Autodesk Inventor part; units mm, degrees
ref_plane "YZ Plane" through (0, 0, 0) normal (1, 0, 0) x (0, 1, 0)
ref_plane "XZ Plane" through (0, 0, 0) normal (0, 1, 0) x (-1, 0, 0)
ref_plane "XY Plane" through (0, 0, 0) normal (0, 0, 1) x (1, 0, 0)
sketch "Sketch1" plane through (0, 0, 0) normal (0, 0, 1) x (1, 0, 0)
  line L0 (3.4641, -6) -> (11.0268, -6)
  line L1 (11.0268, -2) -> (6.0268, -2)
  line L2 (6.0268, -2) -> (6.0268, 2)
  line L3 (6.0268, 2) -> (11.0268, 2)
  line L4 (11.0268, 6) -> (3.4641, 6)
  line L5 (16.0268, 2) -> (16.0268, 6)
  line L6 (16.0268, -6) -> (16.0268, -2)
  line L7 (16.0268, 6) -> (3.4641, 6)
  line L8 (3.4641, 6) -> (0, 0)
  line L9 (0, 0) -> (3.4641, -6)
  line L10 (3.4641, -6) -> (16.0268, -6)
  line L11 (16.0268, 2) -> (6.0268, 2)
  line L12 (6.0268, 2) -> (6.0268, -2)
  line L13 (6.0268, -2) -> (16.0268, -2)
  line L14 (16.0268, 6) -> (16.0268, 2)
  line L15 (16.0268, -2) -> (16.0268, -6)
  point P0 (0, 0)
  dimension "d8" = 10
  dimension "d9" = 10
extrude "Extrusion1" add sketch "Sketch1" along normal blind 10
chamfer "Chamfer2" distance 2 angle 45 4 edges at (16.0268, 4, 10) (16.0268, -4, 10) (16.0268, -4, 0) (16.0268, 4, 0)
sketch "Sketch3" plane through (3.4641, 6, 10) normal (0, 1, 0) x (1, 0, 0)
  line L0 (10.5627, 10) -> (0, 10)
  line L1 (12.5627, 8) -> (12.5627, 2)
  circle A0 centre (7.5627, 5) radius 0.75
  point P0 (-3.4641, 10)
  dimension "d13" = 1.5
  dimension "d14" = 5
  dimension "d15" = 5
extrude "Extrusion2" cut sketch "Sketch3" against normal blind 22.7
pattern_circular "Circular Pattern1" count 3 over 360 about axis through (0, 0, 0) along (0, 0, 1) of "Extrusion1", "Extrusion2"
sketch "Sketch4" plane through (0, 0, 10) normal (0, 0, 1) x (1, 0, 0)
  circle A0 centre (0, 0) radius 0.75
  dimension "d21" = 1.5
extrude "Extrusion3" cut sketch "Sketch4" against normal blind 8
sketch "Sketch5" plane through (0, 0, 10) normal (0, 0, 1) x (1, 0, 0)
  circle A0 centre (0, 0) radius 0.75
  line L0 (-2.8173, -16.8796) -> (3.4641, -6)
  circle A1 centre (4.4641, 7.7321) radius 1.5
  line L1 (0, 0) -> (3.4641, 6)
  line L2 (3.4641, 6) -> (4.4641, 7.7321)
  circle A2 centre (4.4641, 7.7321) radius 4.5
  dimension "d24" = 3
  dimension "d25" = 2
  dimension "d26" = 9
extrude "Extrusion4" add sketch "Sketch5" against normal blind 9 contours A2
pattern_circular "Circular Pattern2" count 3 over 360 about axis through (0, 0, 10) along (0, 0, -1) of "Extrusion4"
fillet "Fillet1" radius 1.5 2 edges at (0.8874, 10.4629, 5.5) (8.6174, 6, 5.5)
pattern_circular "Circular Pattern3" count 3 over 360 about axis through (0, 0, 10) along (0, 0, -1) of "Fillet1"
equation "\"d27\" = d26"
properties part number "Plunger2"
The listing builds one solid part. Answer for the finished solid, in the listing's coordinates (mm). A direction names the side the tool comes from. Round coordinates to 2 decimals unless told otherwise and drop trailing zeros. Loops run counter-clockwise (first coordinate to the right, second up) from the corner with the lowest first, then second, coordinate; pieces in that order, holes last. Notation, with made-up numbers: M 68,37.5 L 79,37.5 A27 ccw 79,58.5 Z; hole C 48.5,-15.5 d8. An arc over 180 degrees is marked long. Return JSON: item names as keys, results as strings.
Q1. Find section B-B, the plane y = 3. Determine the outline of the cut face in (x, z), plus the area to 3 significant figures.
Results list:
{"outline": "M -12.28,1 L -8.66,1 L -8.66,0 L 14.03,0 L 16.03,2 L 16.03,8 L 14.03,10 L -12.28,10 Z; hole C 11.03,5 d1.5", "area": "274 mm2"}
Q2. Which of the six approach directions +Z, -Z, +X, -X, +Y, -Y give full straight-line access (tool end or side, diameter ignored) to faces 1 (the face through (-3.26, 9.65, 4.93)), 2 (the face through (13, 6, 4)), 3 (the face through (-11.42, -7.78, 3.82))?
Results list:
{"face 1": "+Z, -Z", "face 2": "-Z, +X, +Y", "face 3": "-Z, -X"}
Q3. Find the intervals of material crossed by line 1 along Y through (x, z) = (4.5, 4); line 2 along Y through (x, z) = (-2, 8.5); line 3 along X through (y, z) = (7.5, 6), in increasing order. Write a range as from..to.
Results list:
{"line 1": "y = -12.23..-9.23, -6.23..6.23, 9.23..12.23", "line 2": "y = -15.46..-7.46, -5.8..5.8, 7.46..15.46", "line 3": "x = -11.26..-6.64, -2.02..2.98, 5.95..8.96"}
Q4. The mould has two halves that part along X. Classify faces 4 (the face through (15.013, -3.972, 0.986)), 5 (the face through (-2.371, -12.163, 5.287)), 6 (the face through (-10.289, 4.876, 2.779)): released by +X, released by -X, zero draft, split by the parting line, or undercut.
Results list:
{"face 4": "released by +X", "face 5": "undercut", "face 6": "released by -X"}
Q5. Each of these flat-tipped pins is pushed along its axis until it touches: pin 1 Ø1.9 at (x, y) = (4.5, 9.5) entering from -Z; pin 2 Ø2 at (x, z) = (-7, 6) entering from -Y; pin 3 Ø4.5 at (y, z) = (0, 6) entering from +X; pin 4 Ø3 at (x, z) = (13, 3) entering from +Y. Where does it stop, or does it pass through?
Results list:
{"pin 1": "stops at z = 1", "pin 2": "stops at y = -15.04", "pin 3": "stops at x = 16.03", "pin 4": "stops at y = 6"}
Q6. Find section A-A, the plane z = 3.75. State how many separate pieces and enclosed holes the cut face has, plus the area to 3 significant figures.
Results list:
{"separate pieces": "1", "enclosed holes": "4", "area": "490 mm2"}
